```python
from build123d import *

# Parameters (mm, degrees)
SKETCH1_R           = 22.5
SKETCH1_R_2         = 1.5
SKETCH1_R_3         = 5
BOSS_EXTRUDE1_DEPTH = 6
SKETCH4_R           = 8.5
CUT_EXTRUDE2_DEPTH  = 3
SKETCH6_R           = 3.25
CUT_EXTRUDE3_DEPTH  = 2.5
BOSS_EXTRUDE2_DEPTH = 74
SKETCH7_R           = 20.5
CUT_EXTRUDE4_DEPTH  = 4
CHAMFER2_SIZE       = 1


with BuildPart() as part:
    # Sketch1 → Boss-Extrude1 (new body)
    with BuildSketch(Plane(origin=(0, 0, 0), x_dir=(1, 0, 0), z_dir=(0, 1, 0))):
        Circle(SKETCH1_R)
        with Locations((0, 11)):
            Circle(SKETCH1_R_2, mode=Mode.SUBTRACT)
        with Locations((9.526279442, 5.5)):
            Circle(SKETCH1_R_2, mode=Mode.SUBTRACT)
        with Locations((9.526279442, -5.5)):
            Circle(SKETCH1_R_2, mode=Mode.SUBTRACT)
        with Locations((0, -11)):
            Circle(SKETCH1_R_2, mode=Mode.SUBTRACT)
        with Locations((-9.526279442, -5.5)):
            Circle(SKETCH1_R_2, mode=Mode.SUBTRACT)
        with Locations((-9.526279442, 5.5)):
            Circle(SKETCH1_R_2, mode=Mode.SUBTRACT)
        Circle(SKETCH1_R_3, mode=Mode.SUBTRACT)
    extrude(amount=BOSS_EXTRUDE1_DEPTH)

    # Sketch4 → Cut-Extrude2 (cut)
    with BuildSketch(Plane(origin=(0, 6, 0), x_dir=(1, 0, 0), z_dir=(0, 1, 0))):
        Circle(SKETCH4_R)
    extrude(amount=-CUT_EXTRUDE2_DEPTH, mode=Mode.SUBTRACT)

    # Sketch6 → Cut-Extrude3 (cut)
    with BuildSketch(Plane.XZ):
        with Locations((0, 11)):
            Circle(SKETCH6_R)
        with Locations((9.526279442, -5.5)):
            Circle(SKETCH6_R)
        with Locations((-9.526279442, -5.5)):
            Circle(SKETCH6_R)
    extrude(amount=-CUT_EXTRUDE3_DEPTH, mode=Mode.SUBTRACT)

    # Sketch2 → Boss-Extrude2 (add)
    with BuildSketch(Plane(origin=(0, 6, 0), x_dir=(1, 0, 0), z_dir=(0, 1, 0))):
        with BuildLine():
            Line((5.046971379, 18.835553613), (5.823428515, 21.733331092))
            ThreePointArc((5.823428515, 21.733331092), (0, 22.5), (-5.823428515, 21.733331092))
            Line((-5.823428515, 21.733331092), (-5.046971379, 18.835553613))
            ThreePointArc((-5.046971379, 18.835553613), (0, 19.5), (5.046971379, 18.835553613))
        make_face()
        with BuildLine():
            Line((18.835553613, -5.046971379), (21.733331092, -5.823428515))
            ThreePointArc((21.733331092, -5.823428515), (19.485571585, -11.25), (15.909902577, -15.909902577))
            Line((15.909902577, -15.909902577), (13.788582233, -13.788582233))
            ThreePointArc((13.788582233, -13.788582233), (16.887495374, -9.75), (18.835553613, -5.046971379))
        make_face()
        with BuildLine():
            Line((-13.788582233, -13.788582233), (-15.909902577, -15.909902577))
            ThreePointArc((-15.909902577, -15.909902577), (-19.485571585, -11.25), (-21.733331092, -5.823428515))
            Line((-21.733331092, -5.823428515), (-18.835553613, -5.046971379))
            ThreePointArc((-18.835553613, -5.046971379), (-16.887495374, -9.75), (-13.788582233, -13.788582233))
        make_face()
    extrude(amount=BOSS_EXTRUDE2_DEPTH)

    # Sketch7 → Cut-Extrude4 (cut)
    with BuildSketch(Plane(origin=(0, 80, 0), x_dir=(1, 0, 0), z_dir=(0, 1, 0))):
        Circle(SKETCH7_R)
    extrude(amount=-CUT_EXTRUDE4_DEPTH, mode=Mode.SUBTRACT)

    # Chamfer2
    chamfer2_edges = [part.edges().sort_by_distance(p)[0] for p in [
        (-22.5, 0, 0),
        (19.485571585, 80, 11.25),
        (0, 80, -22.5),
        (-19.485571585, 80, 11.25),
    ]]
    chamfer(chamfer2_edges, length=CHAMFER2_SIZE)


solid = part.part
```
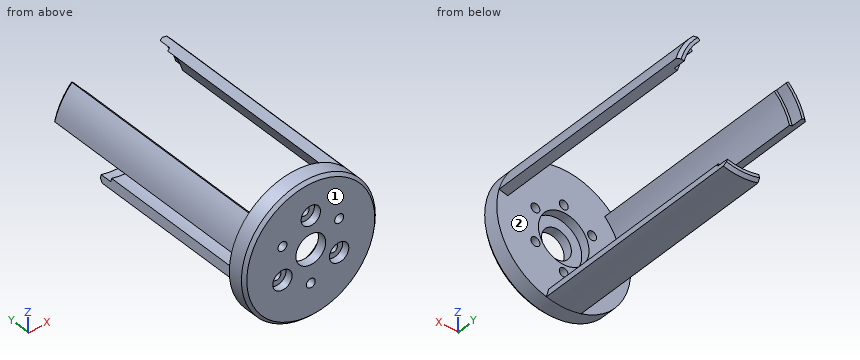
Input: part model. Units: mm. Frame: model coordinates. Face numbers are marked on the shaded views. Coordinates: 2 decimals unless noted, no trailing zeros. Write each loop counter-clockwise with the first axis right and the second up, starting at its lowest first coordinate (ties: lowest second). Pieces come first, ordered by that corner, then holes.
1) Mould query, pull axis X, two halves, no side actions, for the marked faces 1 and 2. Classes: pulls with the +X half, pulls with the -X half, needs draft (parallel to the pull), parting line crosses it, or undercut.
2) Pin query (flat end, axial travel): pin 1 Ø5 at (x, z) = (-9.53, 5.5) entering from +Y; pin 2 Ø13 at (x, z) = (0, 0) entering from +Y; pin 3 Ø6 at (y, z) = (21.5, 4.5) entering from +X; pin 4 Ø2.5 at (x, z) = (9.53, 5.5) entering from +Y. Return the tip coordinate at first contact, or that it passes through.
3) Section A-A on x = 0. State how many separate pieces and enclosed holes the cut face has, and give its area (3 significant figures).
4) Material intervals for line 1 along Z through (x, y) = (0, 1.1); line 2 along X through (y, z) = (1.7, 0); line 3 along Y through (x, z) = (1.5, 18), sorted ascending.
5) Section C-C on y = 46. Output: boundary loops of the cut face in (x, z), and give its area (3 significant figures).
6) Section B-B on z = 0. Output: boundary loops of the cut face in (x, y).
Check result:
1. face 1: needs draft
1. face 2: undercut
2. pin 1: stops at y = 6
2. pin 2: stops at y = 3
2. pin 3: stops at x = 21.73
2. pin 4: passes through
3. separate pieces: 4
3. enclosed holes: 0
3. area: 361 mm2
4. line 1: z = -22.5 to -12.5, -9.5 to -5, 5 to 7.75, 14.25 to 22.5
4. line 2: x = -22.5 to -5, 5 to 22.5
4. line 3: y = 0 to 6
5. outline: (-21.73, 5.82) - (-18.84, 5.05) arc R19.5 cw to (-13.79, 13.79) - (-15.91, 15.91) arc R22.5 ccw to start; (-5.82, -21.73) arc R22.5 ccw to (5.82, -21.73) - (5.05, -18.84) arc R19.5 cw to (-5.05, -18.84) - close; (13.79, 13.79) arc R19.5 cw to (18.84, 5.05) - (21.73, 5.82) arc R22.5 ccw to (15.91, 15.91) - close
5. area: 99.0 mm2
6. outline: (-22.5, 1) - (-21.5, 0) - (-5, 0) - (-5, 3) - (-8.5, 3) - (-8.5, 6) - (-22.5, 6) - close; (5, 0) - (21.5, 0) - (22.5, 1) - (22.5, 6) - (8.5, 6) - (8.5, 3) - (5, 3) - close
